from build123d import *

# Parameters (mm, degrees)
EXTRUDE_1_DEPTH = 3
EXTRUDE_2_DEPTH = 7


with BuildPart() as part:
    # 草图1 → 凸台-拉伸1 (new body)
    with BuildSketch(Plane.XY):
        Polygon((0, 0), (0, -15.25), (-4, -15.25), (-4, -25.25), (0, -25.25), (0, -28.5), (8, -28.5), (8, -36.5), (0, -36.5), (0, -40.5), (38, -40.5), (38, -25.25), (42, -25.25), (42, -15.25), (38, -15.25), (38, -12), (30, -12), (30, -4), (38, -4), (38, 0), align=None)
    extrude(amount=EXTRUDE_1_DEPTH)

    # 草图2 → 凸台-拉伸2 (add)
    with BuildSketch(Plane.XY.offset(3)):
        Polygon((0, 0), (0, -28.5), (8, -28.5), (8, -36.5), (0, -36.5), (0, -40.5), (38, -40.5), (38, -12), (30, -12), (30, -4), (38, -4), (38, 0), align=None)
    extrude(amount=EXTRUDE_2_DEPTH)


solid = part.part
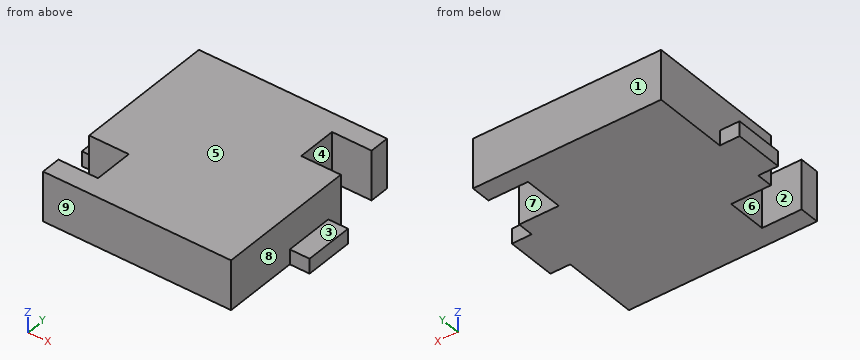
Read the model definition and answer for the solid it produces. Units are mm, in the model's axes. Face numbers are marked on the shaded views. A direction names the side the tool comes from. Round coordinates to 2 decimals unless told otherwise and drop trailing zeros. Loops run counter-clockwise (first coordinate to the right, second up) from the corner with the lowest first, then second, coordinate; pieces in that order, holes last. Notation, with made-up numbers: (-23, 63.5) - (-17, 63.5) arc R31 ccw to (-17, 95.5) - close; hole circle Ø5 at (-3, 34.5). An arc over 180 degrees is marked (long way). One line per question, with ' | ' between items. Start each with the question number.
Q1. Section C-C on y = -23 is taken. Give the vertices of the cut face in (x, z), plus the area to 3 significant figures.
Q2. For a pull along Y with two mould halves and no side action, classify the marked faces 6, 7, 8 and 9 as +Y half, -Y half, draft (parallel to the pull), parting line (faces both ways), or undercut.
Q3. Section D-D on y = -30 is taken. Give the vertices of the cut face in (x, z), plus the area to 3 significant figures.
Q4. Section B-B on z = 9.25 is taken. Give the vertices of the cut face in (x, y).
Q5. Flat-ended cylindrical pins translate along their axes: pin 1 (1.5 mm diameter, centred on y = -35.5, z = 1.5, fed in from +X); pin 2 (0.9 mm diameter, centred on x = 40, z = 1, fed in from +Y); pin 3 (1.5 mm diameter, centred on y = -24.5, z = 6.5, fed in from -X). Find the tip coordinate at first contact, or state that the pin passes through.
Q6. Find the intervals of material crossed by L1, parallel to Y at x = 32, z = 9; L2, parallel to Y at x = 7, z = 8; L3, parallel to X at y = -22, z = 4.75, in increasing order.
Q7. Section A-A on x = 1.5 is taken. Give the vertices of the cut face in (y, z), plus the area to 3 significant figures.
Q8. For the marked faces 1, 2, 3, 4 and 5, determine the directions among +Z, -Z, +X, -X, +Y, -Y from which every point of the face is accessible in a straight line to the end or side of a thin tool.
Established:
1) outline: (-4, 0) - (42, 0) - (42, 3) - (38, 3) - (38, 10) - (0, 10) - (0, 3) - (-4, 3) - close | area: 404 mm²
2) face 6: undercut | face 7: undercut | face 8: draft | face 9: -Y half
3) outline: (8, 0) - (38, 0) - (38, 10) - (8, 10) - close | area: 300 mm²
4) outline: (0, -40.5) - (38, -40.5) - (38, -12) - (30, -12) - (30, -4) - (38, -4) - (38, 0) - (0, 0) - (0, -28.5) - (8, -28.5) - (8, -36.5) - (0, -36.5) - close
5) pin 1: x = 38 | pin 2: y = -15.25 | pin 3: x = 0
6) L1: -40.5 to -12, -4 to 0 | L2: -40.5 to -36.5, -28.5 to 0 | L3: 0 to 38
7) outline: (-40.5, 0) - (-36.5, 0) - (-36.5, 10) - (-40.5, 10) - close; (-28.5, 0) - (0, 0) - (0, 10) - (-28.5, 10) - close | area: 325 mm²
8) face 1: +Z, -Z, +X, -X, +Y | face 2: +Z, -Z, -X | face 3: +Z, +X, +Y, -Y | face 4: +Z, -Z, +X | face 5: +Z, +X, -X, +Y, -Y
